Part model, mm, in its own coordinate system. A direction names the side the tool comes from. Round coordinates to 2 decimals unless told otherwise and drop trailing zeros. Loops run counter-clockwise (first coordinate to the right, second up) from the corner with the lowest first, then second, coordinate; pieces in that order, holes last. Notation, with made-up numbers: M 78,29.25 L 126,29.25 A29 cw 126,66.25 Z; hole C 60,-16 d7. An arc over 180 degrees is marked long. Write each question's results on one line, items separated by ' | '.
Autodesk Inventor part; units mm, degrees
ref_plane "YZ Plane" through (0, 0, 0) normal (1, 0, 0) x (0, 1, 0)
ref_plane "XZ Plane" through (0, 0, 0) normal (0, 1, 0) x (-1, 0, 0)
sketch "Sketch1" plane through (0, 0, 0) normal (0, 0, 1) x (1, 0, 0)
  circle A0 centre (0, 0) radius 6.35
  dimension "d0" = 12.7
extrude "Extrusion1" add sketch "Sketch1" along normal mid plane 63.5
ref_plane "Work Plane1" through (0, 0, 25.4) normal (0, 0, 1) x (1, 0, 0)
sketch "Sketch2" plane through (0, 0, 25.4) normal (0, 0, 1) x (1, 0, 0)
  circle A0 centre (0, 0) radius 6.35
  circle A1 centre (0, 0) radius 6.35
  circle A2 centre (0, 0) radius 5.9436
  dimension "d4" = 12.7
  dimension "d5" = 11.8872
extrude "Extrusion2" cut sketch "Sketch2" against normal blind 0.9906
mirror "Mirror1" about plane through (0, 0, 0) normal (0, 0, 1) of "Extrusion2"
ref_plane "Work Plane2" through (0, 0, -25.4) normal (0, 0, 1) x (1, 0, 0)
properties part number "Linear Actuator Top Scoop Pin .5in. Dia." material "Aluminum 6061"
Item 1: Band-saw the part on C-C on z = -5.5. Give the cut face in (x, y).
Filled sheet:
outline: C 0,0 d12.7
Item 2: Drop flat-ended pins along their axis: P1, Ø1, axis at y = 2.5, z = -11.5, coming from the +X side; P2, Ø3, axis at x = -3.5, z = -16, coming from the -Y side. Give the stop position or say it passes through.
Filled sheet:
P1: x = 6.03 | P2: y = -6.03
Item 3: Band-saw the part on B-B on y = -2.5. Give the cut face in (x, z), and give its area (3 significant figures).
Filled sheet:
outline: M -5.84,-31.75 L 5.84,-31.75 L 5.84,-25.4 L 5.39,-25.4 L 5.39,-24.41 L 5.84,-24.41 L 5.84,24.41 L 5.39,24.41 L 5.39,25.4 L 5.84,25.4 L 5.84,31.75 L -5.84,31.75 L -5.84,25.4 L -5.39,25.4 L -5.39,24.41 L -5.84,24.41 L -5.84,-24.41 L -5.39,-24.41 L -5.39,-25.4 L -5.84,-25.4 Z | area: 740 mm^2
Item 4: Two-plate mould, pull along Z, no slides. Class faces 1 (the flat face through (0, 0, -31.75)), 2 (the cylindrical face through (5.669, 1.785, 24.912)), 3 (the cylindrical face through (-1.38, 6.2, 28.53)): +Z half, -Z half, draft (parallel to the pull), parting line (faces both ways), or undercut.
Filled sheet:
face 1: -Z half | face 2: undercut | face 3: draft
Item 5: Which spindle directions (+Z, -Z, +X, -X, +Y, -Y) get a long thin tool onto all of the face, cutting with end or side? Do faces 4 (the cylindrical face through (-1.38, -6.2, -28.53)), 5 (the cylindrical face through (5.669, -1.785, -24.912)). Say none if no direction does.
Filled sheet:
face 4: +Z, -Z | face 5: none
Item 6: Band-saw the part on A-A on x = 3.25. Give the cut face in (y, z), and give its area (3 significant figures).
Filled sheet:
outline: M -5.46,-31.75 L 5.46,-31.75 L 5.46,-25.4 L 4.98,-25.4 L 4.98,-24.41 L 5.46,-24.41 L 5.46,24.41 L 4.98,24.41 L 4.98,25.4 L 5.46,25.4 L 5.46,31.75 L -5.46,31.75 L -5.46,25.4 L -4.98,25.4 L -4.98,24.41 L -5.46,24.41 L -5.46,-24.41 L -4.98,-24.41 L -4.98,-25.4 L -5.46,-25.4 Z | area: 691 mm^2
Item 7: Wall check: L1, parallel to Z at x = -4, y = -4.75; L2, parallel to Y at x = 0.25, z = -21.5; L3, parallel to X at y = -0.5, z = 17. Give the ranges that are in metal, low to high.
Filled sheet:
L1: -31.75 to -25.4, -24.41 to 24.41, 25.4 to 31.75 | L2: -6.35 to 6.35 | L3: -6.33 to 6.33
